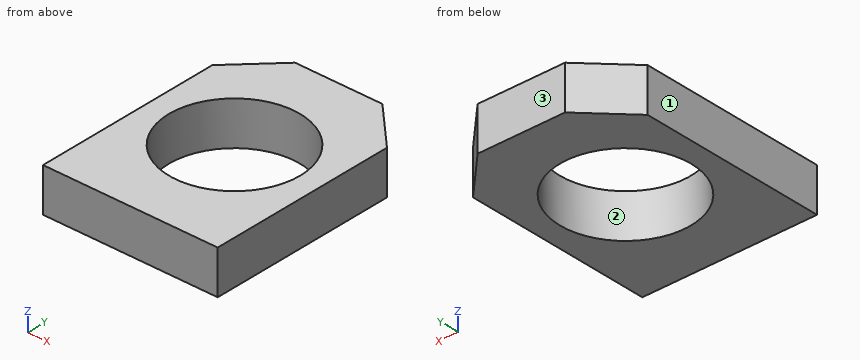
from build123d import *

# Parameters (mm, degrees)
SKETCH1_W           = 38.1
SKETCH1_H           = 9.525
BOSS_EXTRUDE1_DEPTH = 25.4
SKETCH3_R           = 14.2875
CUT_EXTRUDE1_DEPTH  = 34.147973166
CUT_EXTRUDE2_DEPTH  = 34.147973166


with BuildPart() as part:
    # Sketch1 → Boss-Extrude1 (new, symmetric)
    with BuildSketch(Plane(origin=(0, 0, 0), x_dir=(1, 0, 0), z_dir=(0, 1, 0))):
        with Locations((0, -4.7625)):
            Rectangle(SKETCH1_W, SKETCH1_H)
    extrude(amount=BOSS_EXTRUDE1_DEPTH, both=True)

    # Sketch3 → Cut-Extrude1 (cut, through all)
    with BuildSketch(Plane(origin=(0, 0, 0), x_dir=(-1, 0, 0), z_dir=(0, 0, -1))):
        Circle(SKETCH3_R)
    extrude(amount=-CUT_EXTRUDE1_DEPTH, mode=Mode.SUBTRACT)

    # Sketch4 → Cut-Extrude2 (cut, through all)
    with BuildSketch(Plane(origin=(0, 0, 0), x_dir=(-1, 0, 0), z_dir=(0, 0, -1))):
        Polygon((-9.525, 25.4), (-19.05, 15.875), (-19.05, 25.4), align=None)
        Polygon((9.525, 25.4), (19.05, 25.4), (19.05, 15.875), align=None)
    extrude(amount=-CUT_EXTRUDE2_DEPTH, mode=Mode.SUBTRACT)


solid = part.part
Can you work these out from the model? Positions are in its coordinate system, mm. Face numbers are marked on the shaded views. Give positions to 0.01 mm unless a question says otherwise; leave off trailing zeros. Order: outer loops, then holes, each group sorted by start corner. A loop starts at its lowest first (then second) coordinate and runs counter-clockwise, first axis right, second up. Notation, with made-up numbers: M 40,-19 L 84,-19 A12 cw 84,4 Z; hole C 89,-17 d4. An arc over 180 degrees is marked long. One line per item, written item: value.
Item 1: Please list where these lines run through material, in increasing order: line 1 (Y direction, x = 0, z = 7.25); line 2 (Y direction, x = -6, z = 1.25); line 3 (X direction, y = 11, z = 7.25).
Verdict:
line 1: -25.4 to -14.29, 14.29 to 25.4
line 2: -25.4 to -12.97, 12.97 to 25.4
line 3: -19.05 to -9.12, 9.12 to 19.05
Item 2: If we section it at D-D on y = 19.5: Write out the boundary of the cut face in (x, z) (3 decimals), and give its area (3 significant figures).
Verdict:
outline: M -15.425,0 L 15.425,0 L 15.425,9.525 L -15.425,9.525 Z
area: 294 mm2
Item 3: If we section it at C-C on x = 0: Write out the boundary of the cut face in (y, z) (1 decimal), and give its area (3 significant figures).
Verdict:
outline: M -25.4,0 L -14.3,0 L -14.3,9.5 L -25.4,9.5 Z; M 14.3,0 L 25.4,0 L 25.4,9.5 L 14.3,9.5 Z
area: 212 mm2
Item 4: If we mould it in two halves opening along X, with no side actions, what happens to the marked faces 1, 2 and 3? For each: pulls with the +X half, pulls with the -X half, needs draft (parallel to the pull), parting line crosses it, or undercut.
Verdict:
face 1: pulls with the -X half
face 2: undercut
face 3: needs draft
